```python
from build123d import *

# Parameters (mm, degrees)
BOSS_EXTRUDE1_DEPTH = 0.5
CUT_EXTRUDE1_REACH  = 3
SKETCH2_R           = 1.4478


with BuildPart() as part:
    # Sketch1 → Boss-Extrude1 (new body, symmetric)
    with BuildSketch(Plane(origin=(0, 0, 0), x_dir=(1, 0, 0), z_dir=(0, 1, 0))):
        with BuildLine():
            Line((-13.292893219, -2.530330086), (13.292893219, -2.530330086))
            ThreePointArc((13.292893219, -2.530330086), (13.754832985, -2.221671802), (13.646446609, -1.676776695))
            Line((13.646446609, -1.676776695), (10.292893219, 1.676776695))
            ThreePointArc((10.292893219, 1.676776695), (9.96846987, 1.893549447), (9.585786438, 1.969669914))
            Line((9.585786438, 1.969669914), (-9.585786438, 1.969669914))
            ThreePointArc((-9.585786438, 1.969669914), (-9.96846987, 1.893549447), (-10.292893219, 1.676776695))
            Line((-10.292893219, 1.676776695), (-13.646446609, -1.676776695))
            ThreePointArc((-13.646446609, -1.676776695), (-13.754832985, -2.221671802), (-13.292893219, -2.530330086))
        make_face()
    extrude(amount=BOSS_EXTRUDE1_DEPTH, both=True)

    # Sketch2 → Cut-Extrude1 (cut, up to next)
    with BuildSketch(Plane(origin=(0, 0.5, 0), x_dir=(1, 0, 0), z_dir=(0, 1, 0)), mode=Mode.PRIVATE) as cut_extrude1_sk1:
        with Locations((0, -0.280330086)):
            Circle(SKETCH2_R)
    cut_extrude1_tool1 = extrude(cut_extrude1_sk1.sketch, amount=-CUT_EXTRUDE1_REACH, mode=Mode.PRIVATE) & part.part
    add(cut_extrude1_tool1.solids().sort_by_distance((0, 0.5, 0.28033))[0], mode=Mode.SUBTRACT)


solid = part.part
```
The model under review builds one solid part; all positions refer to its coordinate system, in mm. Give positions to 0.01 mm unless a question says otherwise; leave off trailing zeros. Write each loop counter-clockwise with the first axis right and the second up, starting at its lowest first coordinate (ties: lowest second). Pieces come first, ordered by that corner, then holes.
(1) To check wall thickness, follow L1, parallel to Z at x = 0, y = 0.05; L2, parallel to X at y = -0.4, z = 0.7; L3, parallel to X at y = -0.25, z = 1.1. State the ranges of each line that lie inside material, in increasing order.
(2) Consider section B-B, the plane z = 1.35. Give the boundary of the cut face in (x, y).
(3) Consider section A-A, the plane x = 0. Give the boundary of the cut face in (y, z).
(4) Consider section C-C, the plane y = 0.35. Give the boundary of the cut face in (x, z).
(5) Consider section D-D, the plane x = 11.25. Give the boundary of the cut face in (y, z).
(6) The part is to be moulded in two halves that separate along X. For faces 1 (the cylindrical face through (1.381, 0.007, -0.155)), 2 (the flat face through (11.99, 0.01, 0.02)), 3 (the flat face through (-11.95, 0.01, -0.02)), 4 (the flat face through (0, 0.5, 2)), say which applies: released by +X, released by -X, zero draft, split by the parting line, or undercut.
Returned:
1. L1: z = -1.97 to -1.17, 1.73 to 2.53
1. L2: x = -12.67 to -1.39, 1.39 to 12.67
1. L3: x = -13.07 to -1.19, 1.19 to 13.07
2. outline: (-13.32, -0.5) - (-0.98, -0.5) - (-0.98, 0.5) - (-13.32, 0.5) - close; (0.98, -0.5) - (13.32, -0.5) - (13.32, 0.5) - (0.98, 0.5) - close
3. outline: (-0.5, -1.97) - (0.5, -1.97) - (0.5, -1.17) - (-0.5, -1.17) - close; (-0.5, 1.73) - (0.5, 1.73) - (0.5, 2.53) - (-0.5, 2.53) - close
4. outline: (-13.65, 1.68) - (-10.29, -1.68) arc R1 ccw to (-9.59, -1.97) - (9.59, -1.97) arc R1 ccw to (10.29, -1.68) - (13.65, 1.68) arc R0.5 ccw to (13.29, 2.53) - (-13.29, 2.53) arc R0.5 ccw to start; hole circle Ø2.9 at (0, 0.28)
5. outline: (-0.5, -0.72) - (0.5, -0.72) - (0.5, 2.53) - (-0.5, 2.53) - close
6. face 1: undercut
6. face 2: released by +X
6. face 3: released by -X
6. face 4: zero draft
